from build123d import *

# Parameters (mm, degrees)
F0_R     = 3.175
F1_DEPTH = 3.81


with BuildPart() as f1:
    # F0 (on Top) → F1 (new body)
    with BuildSketch(Plane.XY):
        with BuildLine():
            Line((74.725954, 3.459382), (-64.974046, 3.459382))
            ThreePointArc((-64.974046, 3.459382), (-60.483918, 1.59951), (-58.624046, -2.890618))
            ThreePointArc((-58.624046, -2.890618), (-60.483918, -7.380746), (-64.974046, -9.240618))
            Line((-64.974046, -9.240618), (74.725954, -9.240618))
            ThreePointArc((74.725954, -9.240618), (68.375954, -2.890618), (74.725954, 3.459382))
        make_face()
        with BuildLine():
            ThreePointArc((-52.274046, -6.065618), (-55.449046, -2.890618), (-52.274046, 0.284382))
            Line((-52.274046, 0.284382), (62.025954, 0.284382))
            ThreePointArc((62.025954, 0.284382), (64.271018, -0.645554), (65.200954, -2.890618))
            ThreePointArc((65.200954, -2.890618), (64.271018, -5.135682), (62.025954, -6.065618))
            Line((62.025954, -6.065618), (-52.274046, -6.065618))
        make_face(mode=Mode.SUBTRACT)
        with BuildLine():
            ThreePointArc((81.075954, -2.890618), (79.216082, 1.59951), (74.725954, 3.459382))
            ThreePointArc((74.725954, 3.459382), (68.375954, -2.890618), (74.725954, -9.240618))
            ThreePointArc((74.725954, -9.240618), (79.216082, -7.380746), (81.075954, -2.890618))
        make_face()
        with Locations((74.725954, -2.890618)):
            Circle(F0_R, mode=Mode.SUBTRACT)
        with BuildLine():
            ThreePointArc((-58.624046, -2.890618), (-60.483918, 1.59951), (-64.974046, 3.459382))
            ThreePointArc((-64.974046, 3.459382), (-71.324046, -2.890618), (-64.974046, -9.240618))
            ThreePointArc((-64.974046, -9.240618), (-60.483918, -7.380746), (-58.624046, -2.890618))
        make_face()
        with Locations((-64.974046, -2.890618)):
            Circle(F0_R, mode=Mode.SUBTRACT)
    extrude(amount=F1_DEPTH)


solid = f1.part
Can you work these out from the model? Positions are in its coordinate system, mm. A direction names the side the tool comes from. Give positions to 0.01 mm unless a question says otherwise; leave off trailing zeros. Loops run counter-clockwise (first coordinate to the right, second up) from the corner with the lowest first, then second, coordinate; pieces in that order, holes last. Notation, with made-up numbers: (-27, 64.5) - (23, 64.5) arc R25 cw to (23, 81.5) - close; hole circle Ø3 at (10, 41.25). An arc over 180 degrees is marked (long way). Return JSON: item names as keys, results as strings.
1. I want a section at A-A on x = 31.5. Please give me the cut outline in (y, z).
Output values:
{"outline": "(-9.24, 0) - (-6.07, 0) - (-6.07, 3.81) - (-9.24, 3.81) - close; (0.28, 0) - (3.46, 0) - (3.46, 3.81) - (0.28, 3.81) - close"}
2. We'd pull the mould along Y, two halves only. Please class faces 3 (the face through (6, -6.066, 2)), 4 (the face through (6, 3.459, 2)), 5 (the face through (4, 1, 3.81)), 6 (the face through (-71.323, -2.751, 1.878)): +Y half, -Y half, draft (parallel to the pull), parting line (faces both ways), or undercut.
Output values:
{"face 3": "undercut", "face 4": "+Y half", "face 5": "draft", "face 6": "parting line"}
3. For faces 1 (the face through (4, -9.241, 2)), 2 (the face through (4, 0.284, 2)), which set-ups out of +Z, -Z, +X, -X, +Y, -Y let a thin tool reach every point of the face, with its end or its side?
Output values:
{"face 1": "+Z, -Z, +X, -X, -Y", "face 2": "+Z, -Z"}
4. If I drill on line 1 (Y direction, x = -48, z = 1.2); line 2 (X direction, y = -0.5, z = 3); line 3 (X direction, y = -3.5, z = 1), over which ranges is the centre line in solid material (lowest first)?
Output values:
{"line 1": "y = -9.24 to -6.07, 0.28 to 3.46", "line 2": "x = -70.86 to -67.06, -62.88 to -54.36, 64.12 to 72.64, 76.82 to 80.61", "line 3": "x = -71.29 to -68.09, -61.86 to -55.39, 65.14 to 71.61, 77.84 to 81.05"}
5. I want a section at B-B on z = 1.45. Please give me the cut outline in (x, y) (3 decimals), and give its area (3 significant figures).
Output values:
{"outline": "(-64.974, -9.241) - (74.726, -9.241) arc R6.35 ccw to (74.726, 3.459) - (-64.974, 3.459) arc R6.35 ccw to start; hole circle Ø6.35 at (-64.974, -2.891); hole (-52.274, -6.066) - (62.026, -6.066) arc R3.175 ccw to (62.026, 0.284) - (-52.274, 0.284) arc R3.175 ccw to start; hole circle Ø6.35 at (74.726, -2.891)", "area": "1,080 mm²"}
6. I'm going to push flat-ended pins straight in: pin 1 Ø2 at (y, z) = (-1.5, 3) entering from +X; pin 2 Ø5.5 at (x, y) = (-64.97, -2.89) entering from -Z; pin 3 Ø1.5 at (y, z) = (-8, 2.5) entering from +X. Where does each tip first touch, or does it pass through?
Output values:
{"pin 1": "stops at x = 81.06", "pin 2": "passes through", "pin 3": "stops at x = 79.34"}
7. I want a section at C-C on y = -8. Please give me the cut outline in (x, z).
Output values:
{"outline": "(-68.74, 0) - (78.5, 0) - (78.5, 3.81) - (-68.74, 3.81) - close"}
